Verification items for the finished model (mm, model axes). A direction names the side the tool comes from. Give positions to 0.01 mm unless a question says otherwise; leave off trailing zeros. Loops run counter-clockwise (first coordinate to the right, second up) from the corner with the lowest first, then second, coordinate; pieces in that order, holes last. Notation, with made-up numbers: M 89,-12.5 L 105,-12.5 A7 ccw 105,-4.5 Z; hole C 20,-25.75 d1. An arc over 180 degrees is marked long. Use a Markdown table: item, result.
from build123d import *

# Parameters (mm, degrees)
BOSS_EXTRUDE1_DEPTH            = 7.5
SKETCH2_W                      = 10
SKETCH2_H                      = 10
BOSS_EXTRUDE2_DEPTH            = 12
CUT_EXTRUDE1_DEPTH             = 124.51619327
CUT_EXTRUDE1_DEPTH_BACK        = 124.51619327
SKETCH4_W                      = 14
SKETCH4_H                      = 14
BOSS_EXTRUDE3_DEPTH            = 15
SKETCH7_W                      = 14
SKETCH7_H                      = 14
CUT_EXTRUDE2_DEPTH             = 12
M3_CLEARANCE_HOLE1_D           = 3.4
M3_CLEARANCE_HOLE1_CSINK_D     = 3.45
M3_CLEARANCE_HOLE1_CSINK_ANGLE = 90
FILLET1_R                      = 2
FILLET2_R                      = 5


with BuildPart() as part:
    # Sketch1 → Boss-Extrude1 (new, symmetric)
    with BuildSketch(Plane(origin=(0, 0, 0), x_dir=(1, 0, 0), z_dir=(0, 1, 0))):
        Polygon((25, 107.5), (35, 107.5), (35, -117.5), (-35, -117.5), (-35, 107.5), (-25, 107.5), (-25, -107.5), (25, -107.5), align=None)
    extrude(amount=BOSS_EXTRUDE1_DEPTH, both=True)

    # Sketch2 → Boss-Extrude2 (add)
    with BuildSketch(Plane(origin=(0, 0, -107.5), x_dir=(-1, 0, 0), z_dir=(0, 0, -1))):
        with Locations((-30, 12.5)):
            Rectangle(SKETCH2_W, SKETCH2_H)
        Polygon((-35, 21.5), (-35, 17.5), (-25, 17.5), (25, 17.5), (35, 17.5), (35, 21.5), align=None)
        with Locations((30, 12.5)):
            Rectangle(SKETCH2_W, SKETCH2_H)
    extrude(amount=-BOSS_EXTRUDE2_DEPTH)

    # Sketch3 → Cut-Extrude1 (cut, two sides: drawn at the far end of the back side and taken through both)
    with BuildSketch(Plane(origin=(0, 7.5, 0), x_dir=(1, 0, 0), z_dir=(0, 1, 0)).offset(-CUT_EXTRUDE1_DEPTH_BACK)):
        Polygon((-35, -117.5), (35, -117.5), (35, -112.5), (35, 107.5), (32, 107.5), (32, -112.5), (-32, -112.5), (-32, 107.5), (-35, 107.5), (-35, -112.5), align=None)
    extrude(amount=CUT_EXTRUDE1_DEPTH + CUT_EXTRUDE1_DEPTH_BACK, mode=Mode.SUBTRACT)

    # Sketch4 → Boss-Extrude3 (add)
    with BuildSketch(Plane(origin=(0, 7.5, 0), x_dir=(1, 0, 0), z_dir=(0, 1, 0))):
        with Locations((-39, 37)):
            Rectangle(SKETCH4_W, SKETCH4_H)
        with Locations((39, -37)):
            Rectangle(SKETCH4_W, SKETCH4_H)
        with Locations((-39, -37)):
            Rectangle(SKETCH4_W, SKETCH4_H)
        with Locations((39, 37)):
            Rectangle(SKETCH4_W, SKETCH4_H)
    extrude(amount=-BOSS_EXTRUDE3_DEPTH)

    # Sketch7 → Cut-Extrude2 (cut)
    with BuildSketch(Plane(origin=(0, 7.5, 0), x_dir=(1, 0, 0), z_dir=(0, 1, 0))):
        with Locations((-39, 37)):
            Rectangle(SKETCH7_W, SKETCH7_H)
        with Locations((39, 37)):
            Rectangle(SKETCH7_W, SKETCH7_H)
        with Locations((39, -37)):
            Rectangle(SKETCH7_W, SKETCH7_H)
        with Locations((-39, -37)):
            Rectangle(SKETCH7_W, SKETCH7_H)
    extrude(amount=-CUT_EXTRUDE2_DEPTH, mode=Mode.SUBTRACT)

    # M3 Clearance Hole1 (through all)
    with Locations(Plane(origin=(0, -4.5, 0), x_dir=(1, 0, 0), z_dir=(0, 1, 0))):
        with Locations((-39, 37), (39, 37), (39, -37), (-39, -37)):
            CounterSinkHole(M3_CLEARANCE_HOLE1_D / 2, M3_CLEARANCE_HOLE1_CSINK_D / 2, counter_sink_angle=M3_CLEARANCE_HOLE1_CSINK_ANGLE)

    # Fillet1
    fillet1_edges = [part.edges().sort_by_distance(p)[0] for p in [
        (-32, -6, -44),
        (-32, -6, -30),
        (-32, -6, 30),
        (-32, -6, 44),
        (32, -6, 30),
        (32, -6, 44),
        (32, -6, -44),
        (32, -6, -30),
        (-32, -4.5, 37),
        (32, -4.5, 37),
        (32, -4.5, -37),
        (-32, -4.5, -37),
    ]]
    fillet(fillet1_edges, radius=FILLET1_R)

    # Fillet2
    fillet2_edges = [part.edges().sort_by_distance(p)[0] for p in [
        (-46, -6, -30),
        (-46, -6, -44),
        (-46, -6, 44),
        (-46, -6, 30),
        (46, -6, 30),
        (46, -6, 44),
        (46, -6, -44),
        (46, -6, -30),
        (-28.5, 7.5, -95.5),
        (28.5, 7.5, -95.5),
        (-32, 0, 112.5),
        (32, 0, 112.5),
    ]]
    fillet(fillet2_edges, radius=FILLET2_R)


solid = part.part
(1) Cross-section at A-A on x = 10. Record the cut outline in (y, z), then the cut area to 3 significant figures.
Results below:
| item | result |
|---|---|
| outline | M -7.5,107.5 L 7.5,107.5 L 7.5,112.5 L -7.5,112.5 Z; M 17.5,-107.5 L 21.5,-107.5 L 21.5,-95.5 L 17.5,-95.5 Z |
| area | 123 mm^2 |
(2) Gauge pin test, flat ends, axial feed: P1, Ø8, axis at x = -31.5, y = -0.5, coming from the +Z side; P2, Ø7.5, axis at y = 5.5, z = 13, coming from the -X side; P3, Ø1.5, axis at x = -37.5, y = -6, coming from the +Z side; P4, Ø8.5, axis at y = 12, z = 8, coming from the -X side. Record the tip position at first contact, or that the pin passes through.
Results below:
| item | result |
|---|---|
| P1 | z = 112.47 |
| P2 | x = -32 |
| P3 | z = 44 |
| P4 | through |
(3) Cross-section at B-B on z = 84.5. Record the cut outline in (x, y), then the cut area to 3 significant figures.
Results below:
| item | result |
|---|---|
| outline | M -32,-7.5 L -25,-7.5 L -25,7.5 L -32,7.5 Z; M 25,-7.5 L 32,-7.5 L 32,7.5 L 25,7.5 Z |
| area | 210 mm^2 |
(4) Set-up check for faces 1 (the flat face through (-40, -4.5, 35)), 2 (the flat face through (-26, 7.5, 18)), 3 (the flat face through (41, -4.5, -37)): record each of +Z, -Z, +X, -X, +Y, -Y from which the full face is reachable in a straight line by a thin tool's end or side.
Results below:
| item | result |
|---|---|
| face 1 | +Z, -Z, -X, +Y |
| face 2 | +Z, +X, -X, +Y |
| face 3 | +Z, -Z, +X, +Y |
(5) Material ranges on line 1 (Z direction, x = 39, y = -5.45); line 2 (X direction, y = -5.85, z = -37); line 3 (X direction, y = 3.5, z = 94.5), recorded low to high.
Results below:
| item | result |
|---|---|
| line 1 | -44 to -38.7, -35.3 to -30, 30 to 35.3, 38.7 to 44 |
| line 2 | -46 to -40.7, -37.3 to -25, 25 to 37.3, 40.7 to 46 |
| line 3 | -32 to -25, 25 to 32 |
(6) Draft check along Z on faces 4 (the flat face through (-25, -1, -2)), 5 (the cylindrical face through (45, -6, 42)), 6 (the cylindrical face through (-45, -6, -32)). Enter one of: +Z half, -Z half, draft (parallel to the pull), parting line (faces both ways), or undercut.
Results below:
| item | result |
|---|---|
| face 4 | draft |
| face 5 | +Z half |
| face 6 | undercut |
(7) Cross-section at C-C on y = 2.25. Record the cut outline in (x, z), then the cut area to 3 significant figures.
Results below:
| item | result |
|---|---|
| outline | M -32,-107.5 L -25,-107.5 L -25,107.5 L 25,107.5 L 25,-107.5 L 32,-107.5 L 32,107.5 A5 ccw 27,112.5 L -27,112.5 A5 ccw -32,107.5 Z |
| area | 3,320 mm^2 |
